Part model, mm, in its own coordinate system. A direction names the side the tool comes from. Round coordinates to 2 decimals unless told otherwise and drop trailing zeros. Write each loop counter-clockwise with the first axis right and the second up, starting at its lowest first coordinate (ties: lowest second). Pieces come first, ordered by that corner, then holes. Notation, with made-up numbers: (45, -5.75) -> (101, -5.75) arc R31 ccw to (101, 22.25) -> close; hole circle Ø9 at (81.5, -16.75). An arc over 180 degrees is marked (long way). Use CSV: the item, a comma, the result in double quotes. Start each with the question number.
(1) Which spindle directions (+Z, -Z, +X, -X, +Y, -Y) get a long thin tool onto all of the face, cutting with end or side? Do faces 1 (the cylindrical face through (5.77, 25.29, 11.09)), 2 (the flat face through (20, 12, -7)), 3 (the cylindrical face through (14.62, 15.45, -7.09)), 4 (the flat face through (25.422, 15, -27)), 5 (the flat face through (-12.5, 15, -18)). Say none if no direction does.
(2) Two-plate mould, pull along Z, no slides. Class faces 6 (the cylindrical face through (-3.928, 5.916, 21.646)), 7 (the flat face through (6, 19, -22)), 8 (the cylindrical face through (1.802, 16.762, 5.723)): released by +Z, released by -Z, zero draft, split by the parting line, or undercut.
(3) Probe line 1 (X direction, y = 8, z = 0); line 2 (X direction, y = 14, z = 0); line 3 (Y direction, x = -3, z = -27). List the from-to ranges inside material, lowest first. Write a range as [from, to].
(4) Saw through at C-C (z = -21.5). Give the cut face in (x, y), plus the area to 3 significant figures.
(5) Saw through at D-D (x = 14). Give the cut face in (y, z), plus the area to 3 significant figures.
(6) Saw through at B-B (y = 13). Give the cut face in (x, z).
(7) Drop flat-ended pins along their axis: pin 1 (10 mm diameter, centred on y = 27.5, z = 4.5, fed in from +X); pin 2 (3.5 mm diameter, centred on y = 15.5, z = -16, fed in from -X); pin 3 (8 mm diameter, centred on x = 16, z = -3, fed in from -Y); pin 4 (10.5 mm diameter, centred on x = 12, z = -21, fed in from +Y). Give the stop position or say it passes through.
(8) Saw through at A-A (x = 0). Give the cut face in (y, z), plus the area to 4 significant figures.
```python
from build123d import *

# Parameters (mm, degrees)
BOSS_EXTRUDE1_DEPTH = 12
BOSS_EXTRUDE2_DEPTH = 19
SKETCH1_4_R         = 12.5
SKETCH1_4_R_2       = 6
BOSS_EXTRUDE3_DEPTH = 34


with BuildPart() as part:
    # Sketch1 → Boss-Extrude1 (new body)
    with BuildSketch(Plane(origin=(0, 0, 0), x_dir=(1, 0, 0), z_dir=(0, 1, 0))):
        with BuildLine():
            Line((-22, 35), (-22, 0))
            ThreePointArc((-22, 0), (-3.499816256, -21.719836237), (20.886480561, -6.910494177))
            ThreePointArc((20.886480561, -6.910494177), (26.137546313, 0.602202667), (34.650435288, 4))
            ThreePointArc((34.650435288, 4), (54.843960905, 13.995846724), (63, 35))
            Line((63, 35), (25.421858315, 35))
            Line((25.421858315, 35), (25.421858315, 19.331946497))
            ThreePointArc((25.421858315, 19.331946497), (24.072873785, 14.886275206), (20.480860008, 11.939889365))
            ThreePointArc((20.480860008, 11.939889365), (14.678923372, 7.180791818), (12.5, 0))
            ThreePointArc((12.5, 0), (0, -12.5), (-12.5, 0))
            Line((-12.5, 0), (-12.5, 35))
            Line((-12.5, 35), (-22, 35))
        make_face()
    extrude(amount=BOSS_EXTRUDE1_DEPTH)

    # Sketch1_3 → Boss-Extrude2 (add)
    with BuildSketch(Plane(origin=(0, 0, 0), x_dir=(1, 0, 0), z_dir=(0, 1, 0))):
        with BuildLine():
            Line((25.421858315, 35), (-12.5, 35))
            Line((-12.5, 35), (-12.5, 0))
            ThreePointArc((-12.5, 0), (0, 12.5), (12.5, 0))
            ThreePointArc((12.5, 0), (14.678923372, 7.180791818), (20.480860008, 11.939889365))
            ThreePointArc((20.480860008, 11.939889365), (24.072873785, 14.886275206), (25.421858315, 19.331946497))
            Line((25.421858315, 19.331946497), (25.421858315, 35))
        make_face()
    extrude(amount=BOSS_EXTRUDE2_DEPTH)

    # Sketch1_4 → Boss-Extrude3 (add)
    with BuildSketch(Plane(origin=(0, 0, 0), x_dir=(1, 0, 0), z_dir=(0, 1, 0))):
        Circle(SKETCH1_4_R)
        with Locations(Location((0, 0, 0), (0, 0, 270))):
            Circle(SKETCH1_4_R_2, mode=Mode.SUBTRACT)
    extrude(amount=BOSS_EXTRUDE3_DEPTH)


solid = part.part
```
Answers:
1,face 1,"+Y"
1,face 2,"+Z, +Y"
1,face 3,"+Z, +X, +Y"
1,face 4,"+Z, -Z, +X, +Y"
1,face 5,"+Z, -Z, -X, +Y"
2,face 6,"released by +Z"
2,face 7,"zero draft"
2,face 8,"undercut"
3,line 1,"x = [-22, -6], [6, 25.42]"
3,line 2,"x = [-12.5, -6], [6, 12.5]"
3,line 3,"y = [0, 19]"
4,outline,"(-22, 0) -> (59.92, 0) -> (59.92, 12) -> (25.42, 12) -> (25.42, 19) -> (-12.5, 19) -> (-12.5, 12) -> (-22, 12) -> close"
4,area,"1,250 mm²"
5,outline,"(0, -35) -> (19, -35) -> (19, -6.04) -> (12, -6.04) -> (12, 16.97) -> (0, 16.97) -> close"
5,area,"826 mm²"
6,outline,"(-12.5, -35) -> (25.42, -35) -> (25.42, -19.33) arc R8 ccw to (20.48, -11.94) arc R12.92 cw to (12.5, 0) arc R12.5 ccw to (-12.5, 0) -> close; hole circle Ø12 at (0, 0)"
7,pin 1,"stops at x = 12.5"
7,pin 2,"stops at x = -12.5"
7,pin 3,"stops at y = 0"
7,pin 4,"stops at y = 19"
8,outline,"(0, -35) -> (19, -35) -> (19, -12.5) -> (34, -12.5) -> (34, -6) -> (0, -6) -> close; (0, 6) -> (34, 6) -> (34, 12.5) -> (12, 12.5) -> (12, 22) -> (0, 22) -> close"
8,area,"983.5 mm²"
